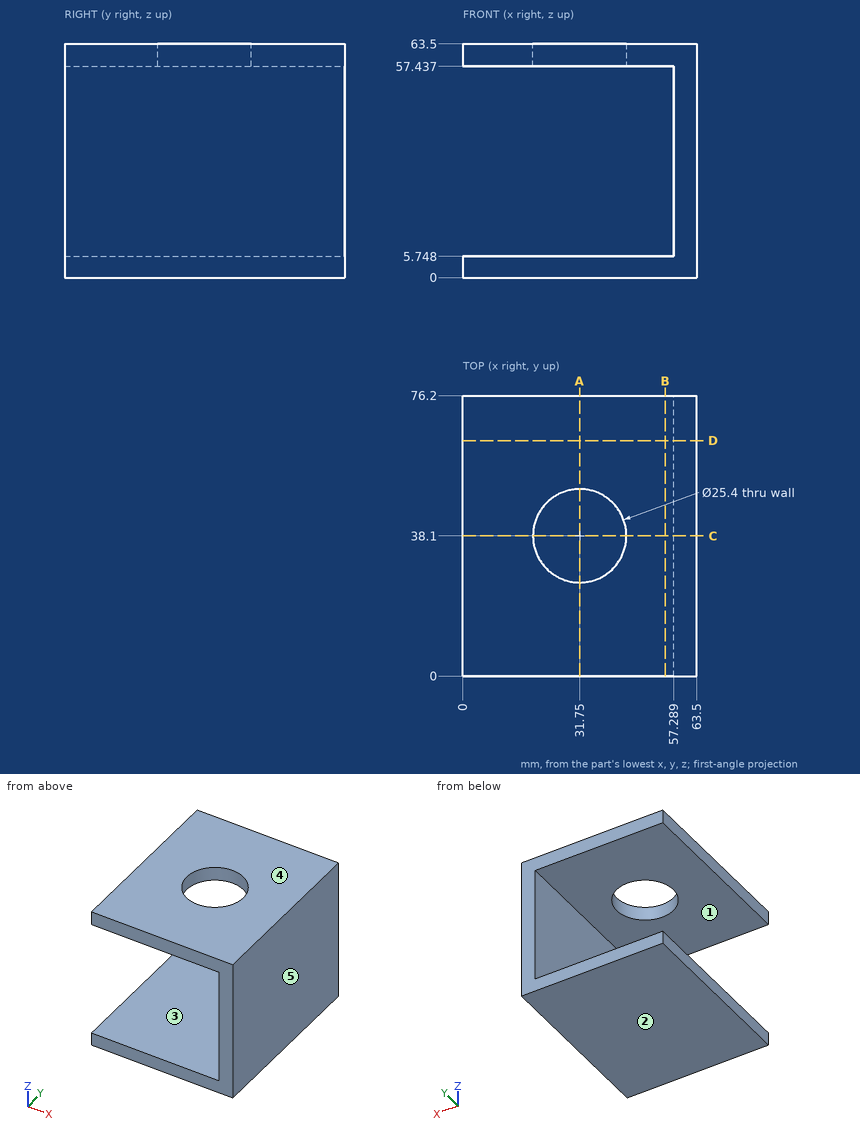
Part print with two shaded views. Sizes in mm from the minimum x, y, z corner. A direction names the side the tool comes from. Round coordinates to 2 decimals unless told otherwise and drop trailing zeros. Order: outer loops, then holes, each group sorted by start corner. A loop starts at its lowest first (then second) coordinate and runs counter-clockwise, first axis right, second up. Notation, with made-up numbers: (82, 7.25) - (90, 7.25) arc R24 ccw to (90, 34.25) - close; hole circle Ø6 at (82.25, 73.25). An arc over 180 degrees is marked (long way). Answer as CSV lines item,"result". Start each with the question number.
1. Drill centre lines: L1, parallel to Z at x = 39, y = 58; L2, parallel to Y at x = 31.75, z = 60.5; L3, parallel to X at y = 38, z = 59. Where is each one in solid material? Low to high. Write a range as [from, to].
2. Tool access for the marked faces 1 and 2: list every direction of +Z, -Z, +X, -X, +Y, -Y with a clear straight run to the whole face (end or side of a thin tool).
3. Pull direction Z, two halves, no side cores. Call the marked faces 3, 4 and 5: +Z half, -Z half, draft (parallel to the pull), parting line (faces both ways), or undercut.
4. Saw through at A-A, the plane x = 31.75. Write the cut outline in (y, z), and give its area (3 significant figures).
5. Pin check, flat tips, straight feed: pin 1 (12 mm diameter, centred on y = 66.5, z = 45, fed in from -X); pin 2 (12 mm diameter, centred on x = 45.5, z = 12.5, fed in from +Y); pin 3 (15 mm diameter, centred on x = 31.75, y = 38.1, fed in from +Z). Stop position of each tip, or through.
6. Saw through at B-B, the plane x = 55. Write the cut outline in (y, z).
7. Saw through at D-D, the plane y = 64. Write the cut outline in (x, z), and give its area (3 significant figures).
8. Saw through at C-C, the plane y = 38.1. Write the cut outline in (x, z), and give its area (3 significant figures).
Model answer:
1,L1,"z = [0, 5.75], [57.44, 63.5]"
1,L2,"y = [0, 25.4], [50.8, 76.2]"
1,L3,"x = [0, 19.05], [44.45, 63.5]"
2,face 1,"-X, +Y, -Y"
2,face 2,"-Z, +X, -X, +Y, -Y"
3,face 3,"undercut"
3,face 4,"+Z half"
3,face 5,"draft"
4,outline,"(0, 0) - (76.2, 0) - (76.2, 5.75) - (0, 5.75) - close; (0, 57.44) - (25.4, 57.44) - (25.4, 63.5) - (0, 63.5) - close; (50.8, 57.44) - (76.2, 57.44) - (76.2, 63.5) - (50.8, 63.5) - close"
4,area,"746 mm²"
5,pin 1,"stops at x = 57.29"
5,pin 2,"passes through"
5,pin 3,"stops at z = 5.75"
6,outline,"(0, 0) - (76.2, 0) - (76.2, 5.75) - (0, 5.75) - close; (0, 57.44) - (76.2, 57.44) - (76.2, 63.5) - (0, 63.5) - close"
7,outline,"(0, 0) - (63.5, 0) - (63.5, 63.5) - (0, 63.5) - (0, 57.44) - (57.29, 57.44) - (57.29, 5.75) - (0, 5.75) - close"
7,area,"1,070 mm²"
8,outline,"(0, 0) - (63.5, 0) - (63.5, 63.5) - (44.45, 63.5) - (44.45, 57.44) - (57.29, 57.44) - (57.29, 5.75) - (0, 5.75) - close; (0, 57.44) - (19.05, 57.44) - (19.05, 63.5) - (0, 63.5) - close"
8,area,"917 mm²"
